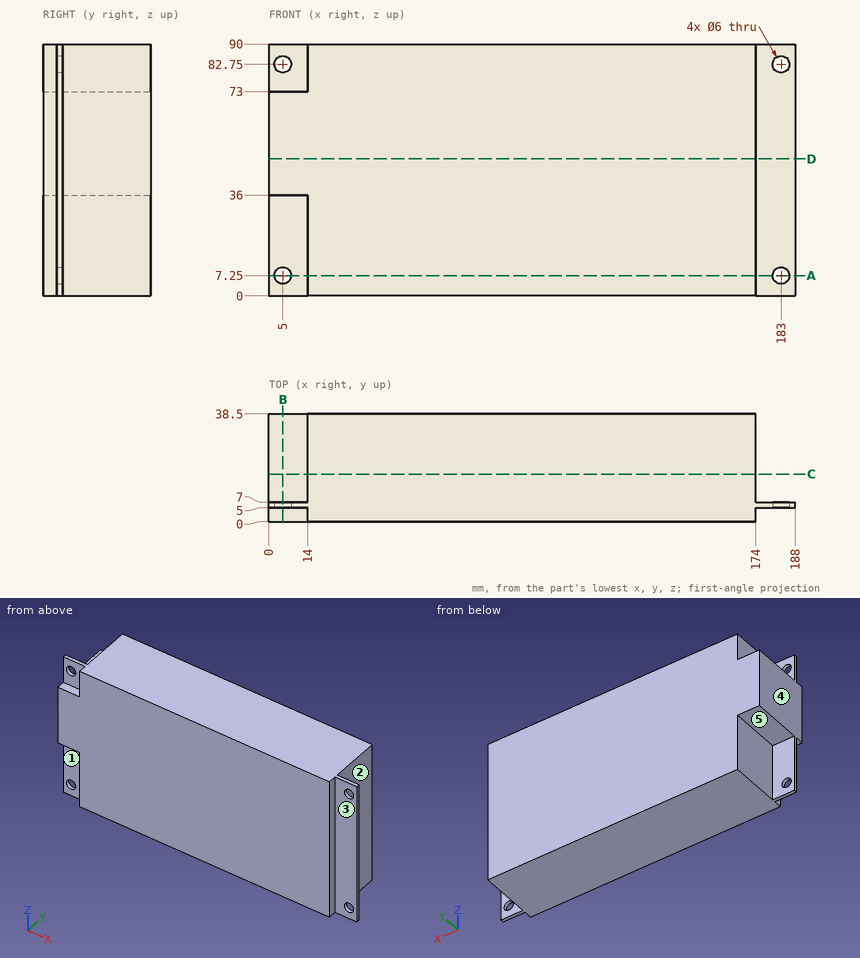
The figure shows three views and two pictorial views of one solid part (mm, origin at its lowest corner). Answer the questions. A direction names the side the tool comes from. Give positions to 0.01 mm unless a question says otherwise; leave off trailing zeros. Order: outer loops, then holes, each group sorted by start corner. A loop starts at its lowest first (then second) coordinate and runs counter-clockwise, first axis right, second up. Notation, with made-up numbers: M 21,-22.75 L 64,-22.75 A16 ccw 64,-8.75 Z; hole C 9.25,-19.75 d2. An arc over 180 degrees is marked long. Return JSON: item names as keys, results as strings.
1) Each of these flat-tipped pins is pushed along its axis until it touches: pin 1 (7 mm diameter, centred on x = 183, z = 7.25, fed in from -Y); pin 2 (8 mm diameter, centred on x = 125, z = 75.5, fed in from -Y); pin 3 (9.5 mm diameter, centred on x = 5, z = 7.25, fed in from +Y); pin 4 (2.5 mm diameter, centred on x = 5.5, y = 2.5, fed in from +Z). Where does it stop, or does it pass through?
Resolved:
{"pin 1": "y = 5", "pin 2": "y = 0", "pin 3": "y = 7", "pin 4": "z = 73"}
2) Section C-C, the plane y = 17 is taken. Write down the section's boundary in (x, z).
Resolved:
{"outline": "M 0,36 L 14,36 L 14,0 L 174,0 L 174,90 L 14,90 L 14,73 L 0,73 Z"}
3) Section D-D, the plane z = 49 is taken. Write down the section's boundary in (x, y).
Resolved:
{"outline": "M 0,0 L 174,0 L 174,5 L 188,5 L 188,7 L 174,7 L 174,38.5 L 0,38.5 Z"}
4) Straight lines are drawn through the part: line 1 along Z through (x, y) = (183, 5.9); line 2 along X through (y, z) = (5.9, 82.75); line 3 along X through (y, z) = (37, 15). For each, find the intervals that lie inside material, in ascending order. Write a range as [from, to].
Resolved:
{"line 1": "[0, 4.25], [10.25, 79.75], [85.75, 90]", "line 2": "[0, 2], [8, 180], [186, 188]", "line 3": "[14, 174]"}
5) Section A-A, the plane z = 7.25 is taken. Write down the section's boundary in (x, y), plus the area to 3 significant figures.
Resolved:
{"outline": "M 0,5 L 2,5 L 2,7 L 0,7 Z; M 8,5 L 14,5 L 14,0 L 174,0 L 174,5 L 180,5 L 180,7 L 174,7 L 174,38.5 L 14,38.5 L 14,7 L 8,7 Z; M 186,5 L 188,5 L 188,7 L 186,7 Z", "area": "6,190 mm^2"}
6) A tool of negligible diameter and unlimited length cuts with its end or side. For the marked faces 1, 2, 3, 4 and 5, from which of +Z, -Z, +X, -X, +Y, -Y can it reach the whole face along a straight path? Write none if from no direction.
Resolved:
{"face 1": "-Z, -X, -Y", "face 2": "+Z, -Z, +X, +Y", "face 3": "+Z, -Z, +X, -Y", "face 4": "+Z, -Z, -X, +Y, -Y", "face 5": "-Z, -X, +Y"}
7) Section B-B, the plane x = 5 is taken. Write down the section's boundary in (y, z), plus the area to 3 significant figures.
Resolved:
{"outline": "M 0,36 L 5,36 L 5,10.25 L 7,10.25 L 7,36 L 38.5,36 L 38.5,73 L 7,73 L 7,79.75 L 5,79.75 L 5,73 L 0,73 Z; M 5,0 L 7,0 L 7,4.25 L 5,4.25 Z; M 5,85.75 L 7,85.75 L 7,90 L 5,90 Z", "area": "1,510 mm^2"}
